Build history of the part. All positions in model axes, mm. Give positions to 0.01 mm unless a question says otherwise; leave off trailing zeros. Order: outer loops, then holes, each group sorted by start corner. A loop starts at its lowest first (then second) coordinate and runs counter-clockwise, first axis right, second up. Notation, with made-up numbers: M 62,41.25 L 71,41.25 A22 ccw 71,79.25 Z; hole C 7,13 d7. An arc over 180 degrees is marked long. One line per item, written item: value. Start each with the question number.
from build123d import *

# Parameters (mm, degrees)
BOSS_EXTRUDE2_DEPTH = 152.4
SKETCH5_W           = 304.8
SKETCH5_H           = 63.5
BOSS_EXTRUDE3_DEPTH = 3.175
BOSS_EXTRUDE4_DEPTH = 3.175


with BuildPart() as part:
    # Sketch4 → Boss-Extrude2 (new body)
    with BuildSketch(Plane(origin=(0, 0, 0), x_dir=(1, 0, 0), z_dir=(0, 1, 0))):
        with BuildLine():
            Line((-149.225, -127), (165.1, -127))
            Line((165.1, -127), (165.1, -130.175))
            Line((165.1, -130.175), (-152.4, -130.175))
            ThreePointArc((-152.4, -130.175), (-156.890128061, -128.315128061), (-158.75, -123.825))
            Line((-158.75, -123.825), (-158.75, 139.7))
            Line((-158.75, 139.7), (-155.575, 139.7))
            Line((-155.575, 139.7), (-155.575, -120.65))
            ThreePointArc((-155.575, -120.65), (-153.715128061, -125.140128061), (-149.225, -127))
        make_face()
    extrude(amount=BOSS_EXTRUDE2_DEPTH)

    # Sketch5 → Boss-Extrude3 (add)
    with BuildSketch(Plane.XY.offset(130.175)):
        with Locations((0, -31.75)):
            Rectangle(SKETCH5_W, SKETCH5_H)
    extrude(amount=-BOSS_EXTRUDE3_DEPTH)

    # Sketch6 → Boss-Extrude4 (add)
    with BuildSketch(Plane.ZY.offset(158.75)):
        with BuildLine():
            Line((-133.35, -180.1876), (-133.35, 0))
            Line((-133.35, 0), (120.65, 0))
            Line((120.65, 0), (120.65, -180.1876))
            Line((120.65, -180.1876), (54.61, -180.1876))
            Line((54.61, -180.1876), (54.61, -139.7))
            ThreePointArc((54.61, -139.7), (-6.35, -78.74), (-67.31, -139.7))
            Line((-67.31, -139.7), (-67.31, -180.1876))
            Line((-67.31, -180.1876), (-133.35, -180.1876))
        make_face()
    extrude(amount=-BOSS_EXTRUDE4_DEPTH)


solid = part.part
1) Drill centre lines: line 1 (X direction, y = -140, z = -96.5) (3 decimals); line 2 (Z direction, x = -118, y = 55.5) (3 decimals). Where is each one in solid material? Low to high.
2) Slice it at B-B (y = 111). List the corners of the cut face in (x, z) (3 decimals).
3) Slice it at D-D (x = -9). List the corners of the cut face in (y, z) (3 decimals).
4) Slice it at A-A (y = -23). List the corners of the cut face in (x, z) (3 decimals).
5) Pull direction Z, two halves, no side cores. Call faces 1 (the cylindrical face through (-157.185, -78.755, -5.01)), 2 (the flat face through (-155.575, 25, -8)), 3 (the flat face through (4, 46, 130.175)): pulls with the +Z half, pulls with the -Z half, needs draft (parallel to the pull), parting line crosses it, or undercut.
6) Drop flat-ended pins along their axis: P1, Ø5, axis at x = -155.5, z = 123.5, coming from the -Y side; P2, Ø5, axis at y = -28.5, z = -22, coming from the +X side (3 decimals); P3, Ø2.5, axis at x = -157, y = -169, coming from the -Z side; P4, Ø3, axis at x = 96.5, y = -65.5, coming from the +Z side. Give the stop position or say it passes through.
7) Slice it at C-C (z = 111). List the corners of the cut face in (x, y) (3 decimals), plus the area to 3 significant figures.
Results list:
1. line 1: x = -158.75 to -155.575
1. line 2: z = 127 to 130.175
2. outline: M -158.75,-139.7 L -155.575,-139.7 L -155.575,120.65 A6.35 cw -149.225,127 L 165.1,127 L 165.1,130.175 L -152.4,130.175 A6.35 ccw -158.75,123.825 Z
3. outline: M -63.5,127 L 152.4,127 L 152.4,130.175 L -63.5,130.175 Z
4. outline: M -158.75,-133.35 L -155.575,-133.35 L -155.575,120.65 L -158.75,120.65 Z; M -152.4,127 L 152.4,127 L 152.4,130.175 L -152.4,130.175 Z
5. face 1: undercut
5. face 2: needs draft
5. face 3: pulls with the +Z half
6. P1: stops at y = 0
6. P2: stops at x = -155.575
6. P3: stops at z = -133.35
6. P4: passes through
7. outline: M -158.75,-180.188 L -155.575,-180.188 L -155.575,152.4 L -158.75,152.4 Z
7. area: 1,060 mm²
